Design review of the part shown in the three views and the two pictorial views. Dimensions are in mm from the part's minimum x, y and z. Round coordinates to 2 decimals unless told otherwise and drop trailing zeros. Write each loop counter-clockwise with the first axis right and the second up, starting at its lowest first coordinate (ties: lowest second). Pieces come first, ordered by that corner, then holes. Notation, with made-up numbers: (9.5, 8) -> (52.5, 8) arc R6 cw to (52.5, 15) -> close; hole circle Ø1 at (55.5, -0.75). An arc over 180 degrees is marked (long way). Return JSON: item names as keys, results as strings. Group by question number.
1. Take a section at C-C, the plane z = 3.6. Give the number of separate pieces and of enclosed holes in the cut face, then the cut area to 3 significant figures.
2. Take a section at D-D, the plane y = 36. Write out the cut boundary in (x, z), then the cut area to 3 significant figures.
3. Take a section at B-B, the plane x = 4. Write out the cut boundary in (y, z), then the cut area to 3 significant figures.
4. For line 1 along Y through (x, z) = (4, 2.1); line 2 along X through (y, z) = (3.5, 1.7); line 3 along X through (y, z) = (33.5, 1.75) (3 decimals), list the stretches that pass through material, from the lowest coordinate up. Write a range as from..to.
5. Mouldability with a two-part tool opening along X and no side actions: class the marked faces 1, 2 and 3 as pulls with the +X half, pulls with the -X half, needs draft (parallel to the pull), parting line crosses it, or undercut.
6. Take a section at A-A, the plane y = 4. Write out the cut boundary in (x, z), then the cut area to 3 significant figures.
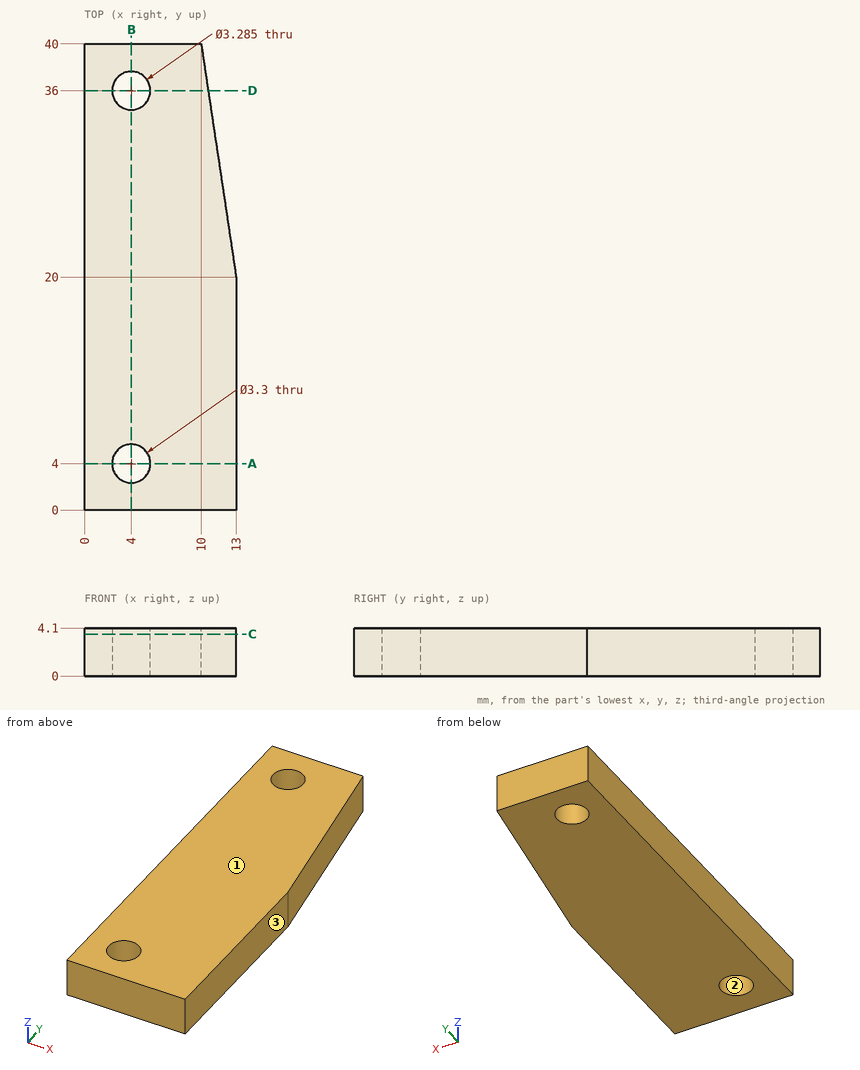
Output:
{
 "1": {"separate pieces": "1", "enclosed holes": "2", "area": "473 mm^2"},
 "2": {"outline": "(0, 0) -> (2.36, 0) -> (2.36, 4.1) -> (0, 4.1) -> close; (5.64, 0) -> (10.6, 0) -> (10.6, 4.1) -> (5.64, 4.1) -> close", "area": "30.0 mm^2"},
 "3": {"outline": "(0, 0) -> (2.35, 0) -> (2.35, 4.1) -> (0, 4.1) -> close; (5.65, 0) -> (34.36, 0) -> (34.36, 4.1) -> (5.65, 4.1) -> close; (37.64, 0) -> (40, 0) -> (40, 4.1) -> (37.64, 4.1) -> close", "area": "137 mm^2"},
 "4": {"line 1": "y = 0..2.35, 5.65..34.36, 37.64..40", "line 2": "x = 0..2.43, 5.57..13", "line 3": "x = 0..10.975"},
 "5": {"face 1": "needs draft", "face 2": "undercut", "face 3": "pulls with the +X half"},
 "6": {"outline": "(0, 0) -> (2.35, 0) -> (2.35, 4.1) -> (0, 4.1) -> close; (5.65, 0) -> (13, 0) -> (13, 4.1) -> (5.65, 4.1) -> close", "area": "39.8 mm^2"}
}
